Build history of the part. All positions in model axes, mm. Face numbers are marked on the shaded views. A direction names the side the tool comes from. Coordinates: 2 decimals unless noted, no trailing zeros. Order: outer loops, then holes, each group sorted by start corner. A loop starts at its lowest first (then second) coordinate and runs counter-clockwise, first axis right, second up. Notation, with made-up numbers: (46.25, 5.25) -> (80.25, 5.25) arc R22 cw to (80.25, 27.25) -> close; hole circle Ø10 at (43.5, 38). An arc over 180 degrees is marked (long way). Write each question's results on one line, items separated by ' | '.
from build123d import *

# Parameters (mm, degrees)
SKETCH1_R               = 5
BOSS_EXTRUDE1_DEPTH     = 8
SKETCH2_R               = 1.6
CUT_EXTRUDE1_DEPTH      = 10
CUT_EXTRUDE2_DEPTH      = 39.34383914
CUT_EXTRUDE2_DEPTH_BACK = 39.34383914


with BuildPart() as part:
    # Sketch1 → Boss-Extrude1 (new body)
    with BuildSketch(Plane.XY):
        with BuildLine():
            Line((0, 0), (-15, 0))
            Line((-15, 0), (-15, 5))
            Line((-15, 5), (-7, 5))
            Line((-7, 5), (-7, 17.5))
            ThreePointArc((-7, 17.5), (-5.535533906, 21.035533906), (-2, 22.5))
            Line((-2, 22.5), (2, 22.5))
            ThreePointArc((2, 22.5), (5.535533906, 21.035533906), (7, 17.5))
            Line((7, 17.5), (7, 5))
            Line((7, 5), (15, 5))
            Line((15, 5), (15, 0))
            Line((15, 0), (0, 0))
        make_face()
        with Locations((0, 14.5)):
            Circle(SKETCH1_R, mode=Mode.SUBTRACT)
    extrude(amount=BOSS_EXTRUDE1_DEPTH)

    # Sketch2 → Cut-Extrude1 (cut)
    with BuildSketch(Plane(origin=(0, 5, 0), x_dir=(1, 0, 0), z_dir=(0, 1, 0))):
        with Locations(Location((-11, -4, 0), (0, 0, 270))):
            Circle(SKETCH2_R)
        with Locations(Location((11, -4, 0), (0, 0, 180))):
            Circle(SKETCH2_R)
    extrude(amount=-CUT_EXTRUDE1_DEPTH, mode=Mode.SUBTRACT)

    # Sketch3 → Cut-Extrude2 (cut, two sides: drawn at the far end of the back side and taken through both)
    with BuildSketch(Plane.ZY.offset(15).offset(-CUT_EXTRUDE2_DEPTH_BACK)):
        Polygon((-12.412584701, -49.305058066), (0, 5), (4, 22.5), (16.412584701, 76.805058066), (-92.197531432, 101.630227468), (-121.022700834, -24.479888665), align=None)
    extrude(amount=CUT_EXTRUDE2_DEPTH + CUT_EXTRUDE2_DEPTH_BACK, mode=Mode.SUBTRACT)


solid = part.part
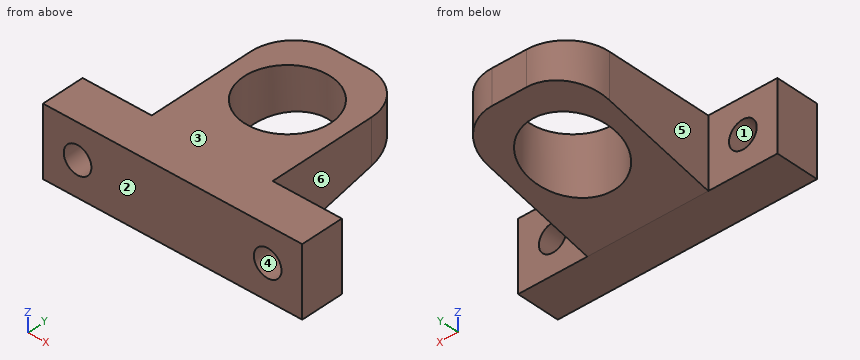
Item 1: Slice it at D-D, the plane z = 6.75. List the corners of the cut face in (x, y), and give its area (3 significant figures).
Answer:
outline: (-15, 0) -> (15, 0) -> (15, 5) -> (7, 5) -> (7, 17.5) arc R5 ccw to (2, 22.5) -> (-2, 22.5) arc R5 ccw to (-7, 17.5) -> (-7, 5) -> (-15, 5) -> close; hole circle Ø10 at (0, 14.5) | area: 306 mm^2
Item 2: Tool access for the marked faces 4, 5 and 6: list every direction of +Z, -Z, +X, -X, +Y, -Y with a clear straight run to the whole face (end or side of a thin tool).
Answer:
face 4: +Y, -Y | face 5: +Z, -Z, -X, +Y | face 6: +Z, -Z, +X, +Y
Item 3: Pin check, flat tips, straight feed: pin 1 (2.5 mm diameter, centred on x = -11.5, z = 2.5, fed in from +Y); pin 2 (3 mm diameter, centred on x = -6, z = 5.5, fed in from +Y); pin 3 (4 mm diameter, centred on x = -1.5, z = 4, fed in from -Y); pin 4 (4 mm diameter, centred on y = 13.5, z = 5.5, fed in from -X). Stop position of each tip, or through.
Answer:
pin 1: stops at y = 5 | pin 2: stops at y = 21.83 | pin 3: stops at y = 0 | pin 4: stops at x = -7
Item 4: Slice it at C-C, the plane y = 13.5. List the corners of the cut face in (x, z).
Answer:
outline: (-7, 1.94) -> (-4.9, 1.94) -> (-4.9, 8) -> (-7, 8) -> close; (4.9, 1.94) -> (7, 1.94) -> (7, 8) -> (4.9, 8) -> close
Item 5: Slice it at B-B, the plane z = 5. List the corners of the cut face in (x, y), and give its area (3 significant figures).
Answer:
outline: (-15, 0) -> (-12.25, 0) -> (-12.25, 5) -> (-15, 5) -> close; (-9.75, 0) -> (9.75, 0) -> (9.75, 5) -> (7, 5) -> (7, 17.5) arc R5 ccw to (2, 22.5) -> (-2, 22.5) arc R5 ccw to (-7, 17.5) -> (-7, 5) -> (-9.75, 5) -> close; (12.25, 0) -> (15, 0) -> (15, 5) -> (12.25, 5) -> close; hole circle Ø10 at (0, 14.5) | area: 281 mm^2
Item 6: Pull direction Z, two halves, no side cores. Call the marked faces 1, 2 and 3: released by +Z, released by -Z, zero draft, split by the parting line, or undercut.
Answer:
face 1: undercut | face 2: zero draft | face 3: released by +Z
Item 7: Drill centre lines: line 1 (X direction, y = 3, z = 4.75); line 2 (X direction, y = 3.5, z = 3); line 3 (Y direction, x = 0, z = 5.25). Where is each one in solid material? Low to high. Write a range as from..to.
Answer:
line 1: x = -15..-12.41, -9.59..9.59, 12.41..15 | line 2: x = -15..-12.25, -9.75..9.75, 12.25..15 | line 3: y = 0..9.5, 19.5..22.5
Item 8: Slice it at A-A, the plane x = 11. List the corners of the cut face in (y, z), and give its area (3 significant figures).
Answer:
outline: (0, 0) -> (5, 0) -> (5, 2.4) -> (0, 2.4) -> close; (0, 5.6) -> (5, 5.6) -> (5, 8) -> (0, 8) -> close | area: 24.0 mm^2
